Autodesk Inventor part; units mm, degrees
ref_plane "YZ Plane" through (0, 0, 0) normal (1, 0, 0) x (0, 1, 0)
ref_plane "XZ Plane" through (0, 0, 0) normal (0, 1, 0) x (-1, 0, 0)
ref_plane "XY Plane" through (0, 0, 0) normal (0, 0, 1) x (1, 0, 0)
sketch "Sketch1" plane through (0, 0, 0) normal (0, 1, 0) x (-1, 0, 0)
  circle A0 centre (0, 0) radius 14.375
  circle A1 centre (0, 0) radius 12
  circle A2 centre (0, 0) radius 13.625
  circle A3 centre (0, 0) radius 12.25
  line L0 (12.25, -5) -> (-12.25, -5)
  line L1 (-12.25, -5) -> (-12.25, 5)
  line L2 (-12.25, 5) -> (12.25, 5)
  line L3 (12.25, 5) -> (12.25, -5)
  line L4 (12.25, -5) -> (-12.25, 5) construction
  line L5 (-12.25, -5) -> (12.25, 5) construction
  point P0 (-10.9087, 5)
  point P1 (-11.1831, 5)
  point P2 (-11.1831, -5)
  point P3 (-10.9087, -5)
  point P4 (11.1831, 5)
  point P5 (10.9087, 5)
  point P6 (10.9087, -5)
  point P7 (11.1831, -5)
  dimension "d0" = 28.75
  dimension "d1" = 24
  dimension "d4" = 27.25
  dimension "d9" = 24.5
  dimension "d10" = 10
extrude "Extrusion1" add sketch "Sketch1" along normal blind 7.5 contours A0 | A1 L2 A3 L0 | A1 L2 A3 | L0 A3 A1 | A1 L0 A3 L2 | L2 L3 A3 | A3 L3 L0 | A3 L1 L2 | L0 L1 A3 | A2
extrude "Extrusion2" cut sketch "Sketch1" along normal blind 2.75 contours A0
thread "Thread1"
extrude "Extrusion3" cut sketch "Sketch1" along normal through all contours A1 L2 A3 L0 | A1 L0 A3 L2
properties part number "Bottom Nut" material "ABS Plastic"
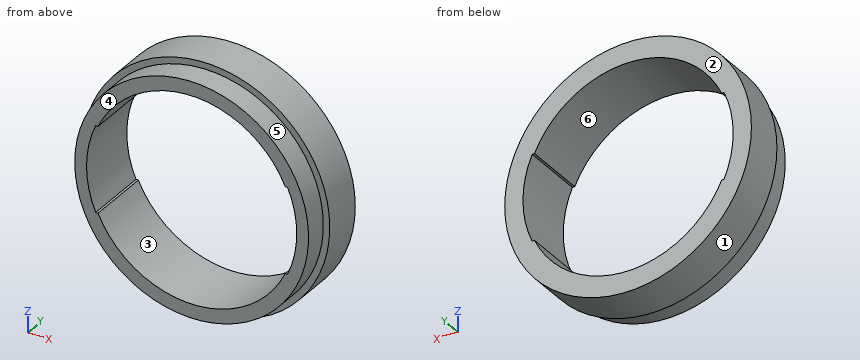
For this review, take the finished solid that the model builds, in its own axes (mm). Face numbers are marked on the shaded views. A direction names the side the tool comes from. Coordinates: 2 decimals unless noted, no trailing zeros. Write each loop counter-clockwise with the first axis right and the second up, starting at its lowest first coordinate (ties: lowest second). Pieces come first, ordered by that corner, then holes. Notation, with made-up numbers: (-7.75, -32) - (13.25, -32) arc R31 ccw to (13.25, 2) - close; hole circle Ø6 at (18, 80.5). An arc over 180 degrees is marked (long way). Answer in a Markdown table with one row per item. Add a question column.
Q1. For probe 1 along Z at (x, y) = (1.5, 6.5); probe 2 along X at (y, z) = (6.75, -6.5); probe 3 along X at (y, z) = (6.5, -9.25), list the stretches that pass through material, from the lowest coordinate up.
Q2. For P1, Ø1.5, axis at y = 2.5, z = 6.5, coming from the -X side; P2, Ø3, axis at y = 4.5, z = -8.5, coming from the +X side; P3, Ø1.5, axis at y = 2.5, z = 11, coming from the -X side, all flat-tipped, find the tip position at first contact; note any pin that passes through.
Q3. Draft analysis for pull direction Z (two halves, no side actions). For the marked faces 1, 2 and 3, state which applies: +Z half, -Z half, draft (parallel to the pull), parting line (faces both ways), or undercut.
Q4. We need section C-C, the plane y = 5.5. State the section outline as (x, z) points (3 decimals).
Q5. We need section A-A, the plane x = 0. State the section outline as (y, z) points (3 decimals).
Q6. Tool access review of the marked faces 4, 5 and 6: name each direction out of +Z, -Z, +X, -X, +Y, -Y from which nothing blocks a thin tool from reaching the whole face with its end or side.
Q7. We need section D-D, the plane y = 1.25. State the section outline as (x, z) points (3 decimals).
Q8. We need section B-B, the plane z = 0. State the section outline as (x, y) points (3 decimals).
Answer list:
| question | item | result |
|---|---|---|
| 1 | probe 1 | z = -14.3 to -11.91, 11.91 to 14.3 |
| 1 | probe 2 | x = -12.82 to -10.09, 10.09 to 12.82 |
| 1 | probe 3 | x = -11 to -7.64, 7.64 to 11 |
| 2 | P1 | stops at x = -13.16 |
| 2 | P2 | stops at x = 12.56 |
| 2 | P3 | stops at x = -10.03 |
| 3 | face 1 | parting line |
| 3 | face 2 | draft |
| 3 | face 3 | undercut |
| 4 | outline | circle Ø28.75 at (0, 0); hole (-11.183, -5) - (-10.909, -5) arc R12 ccw to (10.909, -5) - (11.183, -5) arc R12.25 ccw to (11.183, 5) - (10.909, 5) arc R12 ccw to (-10.909, 5) - (-11.183, 5) arc R12.25 ccw to start |
| 5 | outline | (0, -13.625) - (2.75, -13.625) - (2.75, -14.375) - (7.5, -14.375) - (7.5, -12) - (0, -12) - close; (0, 12) - (7.5, 12) - (7.5, 14.375) - (2.75, 14.375) - (2.75, 13.625) - (0, 13.625) - close |
| 6 | face 4 | +Z, -Z, +X, -X, -Y |
| 6 | face 5 | -Y |
| 6 | face 6 | +Y, -Y |
| 7 | outline | circle Ø27.25 at (0, 0); hole (-11.183, -5) - (-10.909, -5) arc R12 ccw to (10.909, -5) - (11.183, -5) arc R12.25 ccw to (11.183, 5) - (10.909, 5) arc R12 ccw to (-10.909, 5) - (-11.183, 5) arc R12.25 ccw to start |
| 8 | outline | (-14.375, 2.75) - (-13.625, 2.75) - (-13.625, 0) - (-12.25, 0) - (-12.25, 7.5) - (-14.375, 7.5) - close; (12.25, 0) - (13.625, 0) - (13.625, 2.75) - (14.375, 2.75) - (14.375, 7.5) - (12.25, 7.5) - close |
